Verification items for the finished model (mm, model axes). Face numbers are marked on the shaded views. Coordinates: 2 decimals unless noted, no trailing zeros. Order: outer loops, then holes, each group sorted by start corner. A loop starts at its lowest first (then second) coordinate and runs counter-clockwise, first axis right, second up. Notation, with made-up numbers: (35, 84) -> (50, 84) arc R29 ccw to (50, 104) -> close; hole circle Ø1 at (-10, 36). An arc over 180 degrees is marked (long way). Answer as CSV lines item,"result".
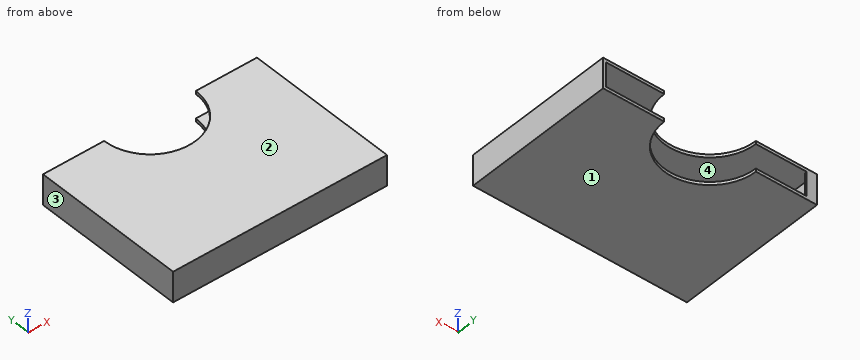
```python
from build123d import *

# Parameters (mm, degrees)
F1_DEPTH = 1.2
F2_DEPTH = 10.5918
F4_DEPTH = 1.2
F6_DEPTH = 9.3918


with BuildPart() as f1:
    # F0 (on Top) → F1 (new body)
    with BuildSketch(Plane.XY):
        with BuildLine():
            Line((-17.78, 58.42), (-40.3225, 58.42))
            Line((-40.3225, 58.42), (-40.3225, 0))
            Line((-40.3225, 0), (40.3225, 0))
            Line((40.3225, 0), (40.3225, 58.42))
            Line((40.3225, 58.42), (17.78, 58.42))
            ThreePointArc((17.78, 58.42), (0, 40.64), (-17.78, 58.42))
        make_face()
        Polygon((-40.3225, 0), (-40.3225, 58.42), (-41.5225, 58.42), (-41.5225, -0.76), (41.5225, -0.76), (41.5225, 58.42), (40.3225, 58.42), (40.3225, 0), align=None)
    extrude(amount=F1_DEPTH)

    # F0 (on Top) → F2 (join)
    with BuildSketch(Plane.XY):
        Polygon((-40.3225, 0), (-40.3225, 58.42), (-41.5225, 58.42), (-41.5225, -0.76), (41.5225, -0.76), (41.5225, 58.42), (40.3225, 58.42), (40.3225, 0), align=None)
    extrude(amount=F2_DEPTH)

    # F3 (on face) → F4 (join)
    with BuildSketch(Plane.XY.offset(10.5918)):
        with BuildLine():
            Line((-40.3225, 58.42), (-41.5225, 58.42))
            Line((-41.5225, 58.42), (-41.5225, -0.76))
            Line((-41.5225, -0.76), (41.5225, -0.76))
            Line((41.5225, -0.76), (41.5225, 58.42))
            Line((41.5225, 58.42), (40.3225, 58.42))
            Line((40.3225, 58.42), (17.78, 58.42))
            ThreePointArc((17.78, 58.42), (0, 40.64), (-17.78, 58.42))
            Line((-17.78, 58.42), (-40.3225, 58.42))
        make_face()
    extrude(amount=F4_DEPTH)

    # F5 (on face) → F6 (join, through all)
    with BuildSketch(Plane.XY.offset(1.2)):
        Polygon((-40.3225, 55.88), (-39.9225, 55.88), (-39.9225, 56.16), (-39.5225, 56.16), (-39.5225, 56.44), (-39.1225, 56.44), (-39.1225, 56.72), (-38.7225, 56.72), (-38.7225, 57), (-38.3225, 57), (-38.3225, 57.28), (-37.9225, 57.28), (-37.9225, 57.56), (-37.5225, 57.56), (-37.5225, 58.42), (-40.3225, 58.42), align=None)
    extrude(amount=F6_DEPTH)


solid = f1.part
```
Item 1: Section check A-A, the plane y = 15. Record the boundary of the cut face in (x, z).
Answer list:
outline,"(-41.52, 0) -> (41.52, 0) -> (41.52, 11.79) -> (-41.52, 11.79) -> close; hole (-40.32, 1.2) -> (40.32, 1.2) -> (40.32, 10.59) -> (-40.32, 10.59) -> close"
Item 2: Section check C-C, the plane x = 0. Record the boundary of the cut face in (y, z).
Answer list:
outline,"(-0.76, 0) -> (40.64, 0) -> (40.64, 1.2) -> (0, 1.2) -> (0, 10.59) -> (40.64, 10.59) -> (40.64, 11.79) -> (-0.76, 11.79) -> close"
Item 3: Release check for a two-part mould opening along Z. For the marked faces 1, 2, 3 and 4 record: +Z half, -Z half, draft (parallel to the pull), parting line (faces both ways), or undercut.
Answer list:
face 1,"-Z half"
face 2,"+Z half"
face 3,"draft"
face 4,"undercut"
Item 4: Thickness scan on line 1 (Z direction, x = 37, y = 45); line 2 (X direction, y = 52, z = 5.75); line 3 (Y direction, x = 16.5, z = 2.75). Record the ranges inside material, lowest first.
Answer list:
line 1,"0 to 1.2, 10.59 to 11.79"
line 2,"-41.52 to -40.32, 40.32 to 41.52"
line 3,"-0.76 to 0"
Item 5: Section check D-D, the plane z = 4.25. Record the boundary of the cut face in (x, y), plus the area to 3 significant figures.
Answer list:
outline,"(-41.52, -0.76) -> (41.52, -0.76) -> (41.52, 58.42) -> (40.32, 58.42) -> (40.32, 0) -> (-40.32, 0) -> (-40.32, 55.88) -> (-39.92, 55.88) -> (-39.92, 56.16) -> (-39.52, 56.16) -> (-39.52, 56.44) -> (-39.12, 56.44) -> (-39.12, 56.72) -> (-38.72, 56.72) -> (-38.72, 57) -> (-38.32, 57) -> (-38.32, 57.28) -> (-37.92, 57.28) -> (-37.92, 57.56) -> (-37.52, 57.56) -> (-37.52, 58.42) -> (-41.52, 58.42) -> close"
area,"208 mm2"
Item 6: Section check B-B, the plane y = 45. Record the boundary of the cut face in (x, z), plus the area to 3 significant figures.
Answer list:
outline,"(-41.52, 0) -> (-11.66, 0) -> (-11.66, 1.2) -> (-40.32, 1.2) -> (-40.32, 10.59) -> (-11.66, 10.59) -> (-11.66, 11.79) -> (-41.52, 11.79) -> close; (11.66, 0) -> (41.52, 0) -> (41.52, 11.79) -> (11.66, 11.79) -> (11.66, 10.59) -> (40.32, 10.59) -> (40.32, 1.2) -> (11.66, 1.2) -> close"
area,"166 mm2"
Item 7: Depth check by flat-ended pin: pin 1 Ø3 at (x, z) = (10, 7.5) entering from +Y. Enter the tip coordinate at first touch or a pass-through.
Answer list:
pin 1,"y = 0"
